```python
from build123d import *

# Parameters (mm, degrees)
PAD_DEPTH       = 3.4
FILLET_R        = 4
SKETCH001_R     = 18
SKETCH001_R_2   = 6.25
PAD001_DEPTH    = 36
SKETCH002_W     = 12
SKETCH002_H     = 42
SKETCH002_R     = 2.65
PAD002_DEPTH    = 48
FILLET002_R     = 2
SKETCH004_W     = 8
SKETCH004_H     = 36.680408
PAD010_DEPTH    = 68
CHAMFER_SIZE    = 20
CHAMFER001_SIZE = 2
SKETCH005_R     = 1.5
POCKET_DEPTH    = 10
SKETCH007_R     = 18
SKETCH007_R_2   = 6.25
PAD012_DEPTH    = 36
SKETCH008_W     = 82.003228
SKETCH008_H     = 66.82692
PAD013_DEPTH    = 3.4
SKETCH009_R     = 3.4
SKETCH009_R_2   = 1.5
PAD014_DEPTH    = 7
FILLET004_R     = 6


with BuildPart() as part:
    # Sketch → Pad (new body)
    with BuildSketch(Plane.XY):
        with BuildLine():
            Line((-65, 0), (-65, -60))
            Line((-65, -60), (65, -60))
            Line((65, -60), (65, 0))
            Line((65, 8), (65, 0))
            ThreePointArc((65, 8), (0, 56.025016), (-65, 8))
            Line((-65, 0), (-65, 8))
        make_face()
    extrude(amount=PAD_DEPTH)

    # Fillet
    fillet_edges = [part.edges().sort_by_distance(p)[0] for p in [
        (65, -60, 1.7),
        (-65, -60, 1.7),
    ]]
    fillet(fillet_edges, radius=FILLET_R)

    # Sketch001 (on Face8 of Pad) → Pad001 (join)
    with BuildSketch(Plane.XY.offset(3.4)):
        with Locations((42, -6)):
            Circle(SKETCH001_R)
        with Locations((42, -6)):
            Circle(SKETCH001_R_2, mode=Mode.SUBTRACT)
    pad001 = extrude(amount=PAD001_DEPTH)

    # Mirrored: Pad001 across YZ
    add(pad001.mirror(Plane.YZ))

    # Sketch002 (on Face5 of Mirrored) → Pad002 (join)
    with BuildSketch(Plane.XY.offset(3.4)):
        with Locations((-27.4, -35)):
            Rectangle(SKETCH002_W, SKETCH002_H)
        with Locations((-27.4, -26)):
            Circle(SKETCH002_R, mode=Mode.SUBTRACT)
        with Locations((-27.4, -44)):
            Circle(SKETCH002_R, mode=Mode.SUBTRACT)
    pad002 = extrude(amount=PAD002_DEPTH)

    # Mirrored001: Pad002 across Sketch002 V_Axis
    add(pad002.mirror(Plane(origin=(0, 0, 3.4), x_dir=(0, 0, 1), z_dir=(1, 0, 0))))

    # Fillet002
    fillet002_edges = [part.edges().sort_by_distance(p)[0] for p in [
        (-33.4, -14, 45.4),
        (33.4, -14, 45.4),
    ]]
    fillet(fillet002_edges, radius=FILLET002_R)

    # Sketch004 (on Face6 of Fillet002) → Pad010 (join)
    with BuildSketch(Plane.XY.offset(3.4)):
        with Locations((37.4, -37.659796)):
            Rectangle(SKETCH004_W, SKETCH004_H)
    extrude(amount=PAD010_DEPTH)

    # Chamfer
    chamfer_edges = [part.edges().sort_by_distance(p)[0] for p in [
        (37.4, -56, 71.4),
    ]]
    chamfer(chamfer_edges, length=CHAMFER_SIZE)

    # Chamfer001
    chamfer001_edges = [part.edges().sort_by_distance(p)[0] for p in [
        (33.4, -46, 61.4),
        (33.4, -27.659796, 71.4),
    ]]
    chamfer(chamfer001_edges, length=CHAMFER001_SIZE)

    # Sketch005 (on Face4 of Chamfer001) → Pocket (cut)
    with BuildSketch(Plane.YZ.offset(41.4)):
        with Locations((-32.7462, 64.451439)):
            Circle(SKETCH005_R)
        with Locations((-22.2462, 64.451439)):
            Circle(SKETCH005_R)
    extrude(amount=-POCKET_DEPTH, mode=Mode.SUBTRACT)

    # Sketch007 (on Face6 of Pocket) → Pad012 (join)
    with BuildSketch(Plane.XY.offset(3.4)):
        with Locations((0, 26)):
            Circle(SKETCH007_R)
        with Locations((0, 26)):
            Circle(SKETCH007_R_2, mode=Mode.SUBTRACT)
    extrude(amount=PAD012_DEPTH)

    # Sketch008 → Pad013 (join)
    with BuildSketch(Plane.XY):
        with Locations((0, -93.41346)):
            Rectangle(SKETCH008_W, SKETCH008_H)
    extrude(amount=PAD013_DEPTH)

    # Sketch009 (on Face21 of Pad013) → Pad014 (join)
    with BuildSketch(Plane.XY.offset(3.4)):
        with Locations((16.9, -119)):
            Circle(SKETCH009_R)
        with Locations((16.9, -119)):
            Circle(SKETCH009_R_2, mode=Mode.SUBTRACT)
        with Locations((-33.9, -103.8)):
            Circle(SKETCH009_R)
        with Locations((-33.9, -103.8)):
            Circle(SKETCH009_R_2, mode=Mode.SUBTRACT)
        with Locations((-33.9, -75.8)):
            Circle(SKETCH009_R)
        with Locations((-33.9, -75.8)):
            Circle(SKETCH009_R_2, mode=Mode.SUBTRACT)
        with Locations((18.2, -70.8)):
            Circle(SKETCH009_R)
        with Locations((18.2, -70.8)):
            Circle(SKETCH009_R_2, mode=Mode.SUBTRACT)
    extrude(amount=PAD014_DEPTH)

    # Fillet004
    fillet004_edges = [part.edges().sort_by_distance(p)[0] for p in [
        (-41.001614, -60, 1.7),
        (41.001614, -60, 1.7),
        (-41.001614, -126.82692, 1.7),
        (41.001614, -126.82692, 1.7),
    ]]
    fillet(fillet004_edges, radius=FILLET004_R)


solid = part.part
```
Could you check a few things on this model? Use its own coordinates, in mm. A direction names the side the tool comes from. Give positions to 0.01 mm unless a question says otherwise; leave off trailing zeros. Loops run counter-clockwise (first coordinate to the right, second up) from the corner with the lowest first, then second, coordinate; pieces in that order, holes last. Notation, with made-up numbers: (6, 14) -> (47, 14) arc R6 ccw to (47, 24) -> close; hole circle Ø5 at (80.5, 3). An arc over 180 degrees is marked (long way). Put each result on its own line as item: value.
(1) Imagine slicing it at D-D on y = 26. Write out the boundary of the cut face in (x, z), plus the area to 3 significant figures.
Computed:
outline: (-56.41, 0) -> (56.41, 0) -> (56.41, 3.4) -> (18, 3.4) -> (18, 39.4) -> (6.25, 39.4) -> (6.25, 3.4) -> (-6.25, 3.4) -> (-6.25, 39.4) -> (-18, 39.4) -> (-18, 3.4) -> (-56.41, 3.4) -> close
area: 1,230 mm^2
(2) For faces 1 (the face through (33.4, -33, 58)), 2 (the face through (63.797, -58.859, 1.724)), 3 (the face through (42, -6, 3.4)), which set-ups out of +Z, -Z, +X, -X, +Y, -Y let a thin tool reach every point of the face, with its end or its side?
Computed:
face 1: +Z, -X, +Y, -Y
face 2: +Z, -Z, +X, -Y
face 3: +Z
(3) Thinking about a two-plate mould opening in Y: for faces 4 (the face through (0, 26, 3.4)), 5 (the face through (-24, -14, 32)), 6 (the face through (-33.2, -77.3, 10.4)), 7 (the face through (-42.806, -61.711, 1.724)), which applies, pulls with the +Y half, pulls with the -Y half, needs draft (parallel to the pull), parting line crosses it, or undercut?
Computed:
face 4: undercut
face 5: undercut
face 6: needs draft
face 7: pulls with the -Y half
(4) Imagine slicing it at A-A on z = 28. State how many separate pieces and enclosed holes the cut face has, plus the area to 3 significant figures.
Computed:
separate pieces: 3
enclosed holes: 7
area: 3,800 mm^2
(5) I'm going to push flat-ended pins straight in: pin 1 Ø5 at (x, z) = (26, 16) entering from +Y; pin 2 Ø3.5 at (x, y) = (17.5, -119.5) entering from +Z; pin 3 Ø10 at (x, y) = (42, -6) entering from -Z; pin 4 Ø5.5 at (y, z) = (-29, 64.5) entering from -X. Where does each tip first touch, or does it pass through?
Computed:
pin 1: y = 5.91
pin 2: z = 10.4
pin 3: z = 0
pin 4: x = 33.4
(6) Please list where these lines run through material, in increasing order: probe 1 along X at (y, z) = (-50, 25); probe 2 along X at (y, z) = (-46, 43.5); probe 3 along Y at (x, z) = (18.2, 7). Write a range as [from, to].
Computed:
probe 1: [-33.4, -21.4], [21.4, 41.4]
probe 2: [-33.4, -29.14], [-25.66, -21.4], [21.4, 25.66], [29.14, 41.4]
probe 3: [-122.14, -119.75], [-118.25, -115.86], [-74.2, -72.3], [-69.3, -67.4]
(7) Imagine slicing it at B-B on y = -26. Write out the boundary of the cut face in (x, z), plus the area to 3 significant figures.
Computed:
outline: (-65, 0) -> (65, 0) -> (65, 3.4) -> (41.4, 3.4) -> (41.4, 71.4) -> (35.4, 71.4) -> (33.4, 69.4) -> (33.4, 51.4) -> (30.05, 51.4) -> (30.05, 3.4) -> (24.75, 3.4) -> (24.75, 51.4) -> (21.4, 51.4) -> (21.4, 3.4) -> (-21.4, 3.4) -> (-21.4, 51.4) -> (-24.75, 51.4) -> (-24.75, 3.4) -> (-30.05, 3.4) -> (-30.05, 51.4) -> (-33.4, 51.4) -> (-33.4, 3.4) -> (-65, 3.4) -> close
area: 1,630 mm^2
